Check sheet for the modelled part. Datum: model origin and axes. Units: mm. A direction names the side the tool comes from. Coordinates: 2 decimals unless noted, no trailing zeros. Write each loop counter-clockwise with the first axis right and the second up, starting at its lowest first coordinate (ties: lowest second). Pieces come first, ordered by that corner, then holes. Notation, with made-up numbers: M -23.5,-37.5 L -2.5,-37.5 A26 ccw -2.5,-23.5 Z; hole C 2,18 d1. An arc over 180 degrees is marked long. Answer as CSV lines item,"result". Start each with the question number.
Q1. Sectioned sample at C-C, the plane z = 19. Record the cut outline in (x, y), then the cut area to 3 significant figures.
Q2. Sectioned sample at A-A, the plane y = 20. Record the cut outline in (x, z), then the cut area to 3 significant figures.
Q3. Thickness scan on line 1 along X through (y, z) = (36.5, -24); line 2 along Y through (x, z) = (36, -56.5); line 3 along X through (y, z) = (16, -23.5). Record the ranges inside material, lowest first. Write a range as from..to.
Q4. Sectioned sample at D-D, the plane z = -56. Record the cut outline in (x, y).
Q5. Sectioned sample at B-B, the plane x = 33.5. Record the cut outline in (y, z).
Q6. Mould release check, pull along Y, two halves, no side actions. Record for faces 5 (the flat face through (11.571, 35, -25)), 6 (the flat face through (37, 30, -25)), 7 (the flat face through (38, 40, -24)): pulls with the +Y half, pulls with the -Y half, needs draft (parallel to the pull), parting line crosses it, or undercut.
Q7. Access from +Z, -Z, +X, -X, +Y, -Y to the whole of each face (thin tool, end or side, straight path). Record for faces 1 (the flat face through (45.071, 20, -25)), 2 (the flat face through (31.571, 35, -25)), 3 (the flat face through (-1.929, 20, -24)), 4 (the flat face through (7, 30, -25)).
Q8. Depth check by flat-ended pin: pin 1 Ø11 at (y, z) = (34, -39) entering from -X; pin 2 Ø3 at (x, z) = (22.5, -48) entering from +Y; pin 3 Ø6 at (x, y) = (-4, 33) entering from -Z. Enter the tip coordinate at first touch or a pass-through.
Autodesk Inventor part; units mm, degrees
ref_plane "YZ Plane" through (0, 0, 0) normal (1, 0, 0) x (0, 1, 0)
ref_plane "XZ Plane" through (0, 0, 0) normal (0, 1, 0) x (-1, 0, 0)
ref_plane "XY Plane" through (0, 0, 0) normal (0, 0, 1) x (1, 0, 0)
sketch "Sketch1" plane through (0, 0, 0) normal (0, 1, 0) x (-1, 0, 0)
  point P0 (0, 0)
sketch "Sketch2" plane through (0, 0, 0) normal (0, 1, 0) x (-1, 0, 0)
  line L0 (10.9292, 17.7027) -> (-54.0708, 17.7027)
  line L1 (-54.0708, 17.7027) -> (-54.0708, -67.2973)
  line L2 (-54.0708, -67.2973) -> (10.9292, -67.2973)
  line L3 (10.9292, -67.2973) -> (10.9292, 17.7027)
  line L4 (10.9292, -24.7973) -> (-21.5708, -24.7973) construction
  line L5 (-21.5708, -24.7973) -> (-21.5708, 9.2027) construction
  line L6 (-21.5708, 9.2027) -> (1.9292, 9.2027)
  line L7 (1.9292, 9.2027) -> (1.9292, -58.7973)
  line L8 (1.9292, -58.7973) -> (-45.0708, -58.7973)
  line L9 (-45.0708, -58.7973) -> (-45.0708, 9.2027)
  line L10 (-45.0708, 9.2027) -> (-21.5708, 9.2027)
  line L11 (10.9292, 12.7027) -> (5.9292, 12.7027) construction
  circle A0 centre (5.9292, 12.7027) radius 3
  line L12 (10.9292, -62.2973) -> (5.9292, -62.2973) construction
  circle A1 centre (5.9292, -62.2973) radius 3
  line L13 (-54.0708, -62.2973) -> (-49.0708, -62.2973) construction
  circle A2 centre (-49.0708, -62.2973) radius 3
  line L14 (-54.0708, 12.7027) -> (-49.0708, 12.7027) construction
  circle A3 centre (-49.0708, 12.7027) radius 3
  point P0 (0, 0)
  dimension "d0" = 65
  dimension "d1" = 85
  dimension "d2" = 34
  dimension "d3" = 23.5
  dimension "d4" = 68
  dimension "d5" = 47
  dimension "d6" = 68
  dimension "d8" = 5
  dimension "d9" = 6
  dimension "d11" = 5
  dimension "d12" = 6
  dimension "d14" = 5
  dimension "d15" = 6
  dimension "d17" = 5
  dimension "d18" = 6
extrude "Extrusion1" add sketch "Sketch2" along normal blind 10 contours L3 L2 L1 L0 | L6 L7 L8 L9 L10
extrude "Extrusion2" cut sketch "Sketch2" along normal blind 20 contours L6 L7 L8 L9 L10
extrude "Extrusion3" add sketch "Sketch2" along normal blind 40 contours L6 L7 L8 L9 L10
sketch "Sketch3" plane through (45.0708, 10, -58.7973) normal (0, 0, -1) x (-1, 0, 0)
  line L0 (47, 30) -> (0, 30)
  line L1 (0, 30) -> (13.5, 30) construction
  line L2 (47, 30) -> (33.5, 30) construction
  line L3 (13.5, 30) -> (13.5, 20)
  line L4 (13.5, 20) -> (3.5, 20)
  line L5 (3.5, 20) -> (3.5, 5)
  line L6 (3.5, 5) -> (43.5, 5)
  line L7 (43.5, 5) -> (43.5, 20)
  line L8 (43.5, 20) -> (33.5, 20)
  line L9 (33.5, 20) -> (33.5, 30)
  line L10 (13.5, 30) -> (33.5, 30)
  point P0 (45.0708, -10)
  dimension "d25" = 13.5
  dimension "d26" = 13.5
  dimension "d27" = 10
  dimension "d28" = 10
  dimension "d29" = 15
  dimension "d30" = 40
  dimension "d31" = 15
  dimension "d32" = 10
extrude "Extrusion4" cut sketch "Sketch3" against normal blind 68
sketch "Sketch4" plane through (45.0708, 10, -58.7973) normal (0, 0, -1) x (-1, 0, 0)
  point P0 (45.0708, -10)
sketch "Sketch5" plane through (0, 0, 0) normal (0, -1, 0) x (1, 0, 0)
  line L0 (-10.9292, 17.7027) -> (54.0708, 17.7027)
  line L1 (-20.9292, 27.7027) -> (64.0708, 27.7027)
  line L2 (64.0708, 27.7027) -> (64.0708, -77.2973)
  line L3 (64.0708, -77.2973) -> (-20.9292, -77.2973)
  line L4 (-20.9292, -77.2973) -> (-20.9292, 27.7027)
  circle A0 centre (54.0708, 17.7027) radius 3
  circle A1 centre (-10.9292, 17.7027) radius 3
  line L5 (54.0708, -67.2973) -> (-10.9292, -67.2973)
  circle A2 centre (-10.9292, -67.2973) radius 3
  circle A3 centre (54.0708, -67.2973) radius 3
  point P0 (0, 0)
  dimension "d37" = 85
  dimension "d38" = 105
  dimension "d41" = 6
  dimension "d42" = 105
  dimension "d43" = 6
  dimension "d44" = 6
  dimension "d45" = 6
extrude "Extrusion5" cut sketch "Sketch2" along normal blind 10
extrude "Extrusion6" add sketch "Sketch5" along normal blind 10
properties part number "Base"
Output:
1,outline,"M -20.93,-10 L -13.63,-10 L -13.63,0 L -20.93,0 Z; M -8.22,-10 L 51.37,-10 L 51.37,0 L -8.22,0 Z; M 56.78,-10 L 64.07,-10 L 64.07,0 L 56.78,0 Z"
1,area,"742 mm^2"
2,outline,"M -1.93,-58.8 L 1.57,-58.8 L 1.57,9.2 L -1.93,9.2 Z; M 41.57,-58.8 L 45.07,-58.8 L 45.07,9.2 L 41.57,9.2 Z"
2,area,"476 mm^2"
3,line 1,"x = -1.93..11.57, 31.57..45.07"
3,line 2,"y = -10..15, 30..40"
3,line 3,"x = -1.93..1.57, 41.57..45.07"
4,outline,"M -20.93,-10 L 64.07,-10 L 64.07,0 L 45.07,0 L 45.07,40 L 31.57,40 L 31.57,30 L 41.57,30 L 41.57,15 L 1.57,15 L 1.57,30 L 11.57,30 L 11.57,40 L -1.93,40 L -1.93,0 L -20.93,0 Z"
5,outline,"M -10,-77.3 L 0,-77.3 L 0,-58.8 L 15,-58.8 L 15,9.2 L 0,9.2 L 0,27.7 L -10,27.7 Z; M 30,-58.8 L 40,-58.8 L 40,9.2 L 30,9.2 Z"
6,face 5,"needs draft"
6,face 6,"undercut"
6,face 7,"pulls with the +Y half"
7,face 1,"+Z, -Z, +X, +Y"
7,face 2,"+Z, -Z, +Y"
7,face 3,"+Z, -Z, -X, +Y"
7,face 4,"+Z, -Z"
8,pin 1,"stops at x = -1.93"
8,pin 2,"stops at y = 15"
8,pin 3,"stops at z = -58.8"
